For this review, take the finished solid that the model builds, in its own axes (mm). Face numbers are marked on the shaded views. A direction names the side the tool comes from. Coordinates: 2 decimals unless noted, no trailing zeros. Order: outer loops, then holes, each group sorted by start corner. A loop starts at its lowest first (then second) coordinate and runs counter-clockwise, first axis right, second up. Notation, with made-up numbers: (76.25, -15) -> (127.25, -15) arc R31 ccw to (127.25, 12) -> close; hole circle Ø3 at (25.5, 46). An arc over 180 degrees is marked (long way). Write item = value, one per line. Start each with the question number.
1) Machinability: for the marked faces 4 and 5, which of the approach directions +Z, -Z, +X, -X, +Y, -Y give a long, thin tool a straight path to every point of the face, cutting with its end or side? Answer none if there is none.
2) Consider section B-B on y = 24.5. Give the boundary of the cut face in (x, z).
3) Consider section C-C on x = -18.5. Give the boundary of the cut face in (y, z), and give its area (3 significant figures).
4) Insertion check: pin 1 Ø3.5 at (x, y) = (39.5, -24.5) entering from -Z. The pin has a flat end and moves straight along its axis. Give the tip position at first contact, or say it passes through.
5) Consider section A-A on x = 39.5. Give the boundary of the cut face in (y, z), and give its area (3 significant figures).
6) Draft analysis for pull direction Y (two halves, no side actions). For the marked faces 1, 2 and 3, state which applies: +Y half, -Y half, draft (parallel to the pull), parting line (faces both ways), or undercut.
7) Wall thickness on probe 1 along Y at (x, z) = (39.5, 11.05); probe 2 along Y at (x, z) = (7.5, 5.5); probe 3 along X at (y, z) = (-20, 9.5): over which ranges is each line inside the solid? List them lowest first. Write a range as [from, to].
8) Consider section D-D on z = 11.5. Give the boundary of the cut face in (x, y).
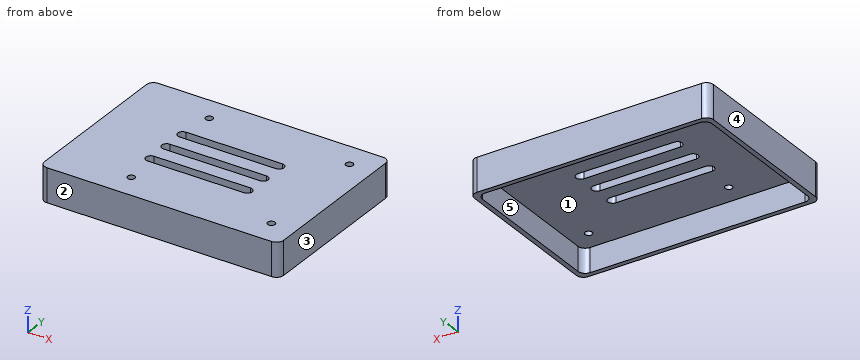
from build123d import *

# Parameters (mm, degrees)
BOSS_EXTRU_1_DEPTH      = 10
BOSS_EXTRU_2_START      = 10
BOSS_EXTRU_2_DEPTH      = 4
ESQUISSE3_R             = 1.5
ENL_V_MAT_EXTRU_1_DEPTH = 63.219369974
ENL_V_MAT_EXTRU_2_DEPTH = 5


with BuildPart() as part:
    # Esquisse1 → Boss.-Extru.1 (new body)
    with BuildSketch(Plane.XY):
        with BuildLine():
            Line((-46.5, -35), (46.5, -35))
            ThreePointArc((46.5, -35), (48.621320344, -34.121320344), (49.5, -32))
            Line((49.5, -32), (49.5, 32))
            ThreePointArc((49.5, 32), (48.621320344, 34.121320344), (46.5, 35))
            Line((46.5, 35), (-46.5, 35))
            ThreePointArc((-46.5, 35), (-48.621320344, 34.121320344), (-49.5, 32))
            Line((-49.5, 32), (-49.5, -32))
            ThreePointArc((-49.5, -32), (-48.621320344, -34.121320344), (-46.5, -35))
        make_face()
        with BuildLine():
            ThreePointArc((44.5, -33), (46.621320344, -32.121320344), (47.5, -30))
            Line((47.5, -30), (47.5, 30))
            ThreePointArc((47.5, 30), (46.621320344, 32.121320344), (44.5, 33))
            Line((44.5, 33), (-44.5, 33))
            ThreePointArc((-44.5, 33), (-46.621320344, 32.121320344), (-47.5, 30))
            Line((-47.5, 30), (-47.5, -30))
            ThreePointArc((-47.5, -30), (-46.621320344, -32.121320344), (-44.5, -33))
            Line((-44.5, -33), (44.5, -33))
        make_face(mode=Mode.SUBTRACT)
    extrude(amount=BOSS_EXTRU_1_DEPTH)

    # Esquisse2 → Boss.-Extru.2 (add)
    with BuildSketch(Plane.XY.offset(BOSS_EXTRU_2_START)):
        with BuildLine():
            Line((-46.5, -35), (46.5, -35))
            ThreePointArc((46.5, -35), (48.621320344, -34.121320344), (49.5, -32))
            Line((49.5, -32), (49.5, 32))
            ThreePointArc((49.5, 32), (48.621320344, 34.121320344), (46.5, 35))
            Line((46.5, 35), (-46.5, 35))
            ThreePointArc((-46.5, 35), (-48.621320344, 34.121320344), (-49.5, 32))
            Line((-49.5, 32), (-49.5, -32))
            ThreePointArc((-49.5, -32), (-48.621320344, -34.121320344), (-46.5, -35))
        make_face()
    extrude(amount=BOSS_EXTRU_2_DEPTH)

    # Esquisse3 → Enlèv. mat.-Extru.1 (cut, through all)
    with BuildSketch(Plane.XY.offset(14)):
        with Locations((39.5, 24.5)):
            Circle(ESQUISSE3_R)
        with Locations((-18.5, 24.5)):
            Circle(ESQUISSE3_R)
        with Locations((39.5, -24.5)):
            Circle(ESQUISSE3_R)
        with Locations((-18.5, -24.5)):
            Circle(ESQUISSE3_R)
    extrude(amount=-ENL_V_MAT_EXTRU_1_DEPTH, mode=Mode.SUBTRACT)

    # Esquisse4 → Enlèv. mat.-Extru.2 (cut)
    with BuildSketch(Plane.XY.offset(14)):
        with BuildLine():
            Line((20, -2), (-20, -2))
            ThreePointArc((-20, -2), (-22, 0), (-20, 2))
            Line((-20, 2), (20, 2))
            ThreePointArc((20, 2), (22, 0), (20, -2))
        make_face()
        with BuildLine():
            Line((20, -12), (-20, -12))
            ThreePointArc((-20, -12), (-22, -10), (-20, -8))
            Line((-20, -8), (20, -8))
            ThreePointArc((20, -8), (22, -10), (20, -12))
        make_face()
        with BuildLine():
            Line((20, 8), (-20, 8))
            ThreePointArc((-20, 8), (-22, 10), (-20, 12))
            Line((-20, 12), (20, 12))
            ThreePointArc((20, 12), (22, 10), (20, 8))
        make_face()
    extrude(amount=-ENL_V_MAT_EXTRU_2_DEPTH, mode=Mode.SUBTRACT)


solid = part.part
Answer sheet:
q1.face_4 = +Z, -Z, -X, +Y, -Y
q1.face_5 = -Z
q2.outline = (-49.5, 0) -> (-47.5, 0) -> (-47.5, 10) -> (-20, 10) -> (-20, 14) -> (-49.5, 14) -> close; (-17, 10) -> (38, 10) -> (38, 14) -> (-17, 14) -> close; (41, 10) -> (47.5, 10) -> (47.5, 0) -> (49.5, 0) -> (49.5, 14) -> (41, 14) -> close
q3.outline = (-35, 0) -> (-33, 0) -> (-33, 10) -> (-26, 10) -> (-26, 14) -> (-35, 14) -> close; (-23, 10) -> (-12, 10) -> (-12, 14) -> (-23, 14) -> close; (-8, 10) -> (-2, 10) -> (-2, 14) -> (-8, 14) -> close; (2, 10) -> (8, 10) -> (8, 14) -> (2, 14) -> close; (12, 10) -> (23, 10) -> (23, 14) -> (12, 14) -> close; (26, 10) -> (33, 10) -> (33, 0) -> (35, 0) -> (35, 14) -> (26, 14) -> close
q3.area = 248 mm2
q4.pin_1 = 10
q5.outline = (-35, 0) -> (-33, 0) -> (-33, 10) -> (-26, 10) -> (-26, 14) -> (-35, 14) -> close; (-23, 10) -> (23, 10) -> (23, 14) -> (-23, 14) -> close; (26, 10) -> (33, 10) -> (33, 0) -> (35, 0) -> (35, 14) -> (26, 14) -> close
q5.area = 296 mm2
q6.face_1 = undercut
q6.face_2 = -Y half
q6.face_3 = draft
q7.probe_1 = [-35, -26], [-23, 23], [26, 35]
q7.probe_2 = [-35, -33], [33, 35]
q7.probe_3 = [-49.5, -47.5], [47.5, 49.5]
q8.outline = (-49.5, -32) arc R3 ccw to (-46.5, -35) -> (46.5, -35) arc R3 ccw to (49.5, -32) -> (49.5, 32) arc R3 ccw to (46.5, 35) -> (-46.5, 35) arc R3 ccw to (-49.5, 32) -> close; hole circle Ø3 at (-18.5, -24.5); hole (-20, -12) -> (20, -12) arc R2 ccw to (20, -8) -> (-20, -8) arc R2 ccw to start; hole (-20, -2) -> (20, -2) arc R2 ccw to (20, 2) -> (-20, 2) arc R2 ccw to start; hole (-20, 8) -> (20, 8) arc R2 ccw to (20, 12) -> (-20, 12) arc R2 ccw to start; hole circle Ø3 at (-18.5, 24.5); hole circle Ø3 at (39.5, -24.5); hole circle Ø3 at (39.5, 24.5)
